Answer from the drawing. Dimensions are ordinates in mm from the lowest x, y and z of the part. Give positions to 0.01 mm unless a question says otherwise; leave off trailing zeros. Write each loop counter-clockwise with the first axis right and the second up, starting at its lowest first coordinate (ties: lowest second). Pieces come first, ordered by that corner, then holes. Notation, with made-up numbers: (-28.5, 29.5) - (29.5, 29.5) arc R28 cw to (29.5, 48.5) - close; hole circle Ø9 at (78.5, 83). An arc over 180 degrees is marked (long way). Answer as a JSON object with one key per item and string values. Group by question number.
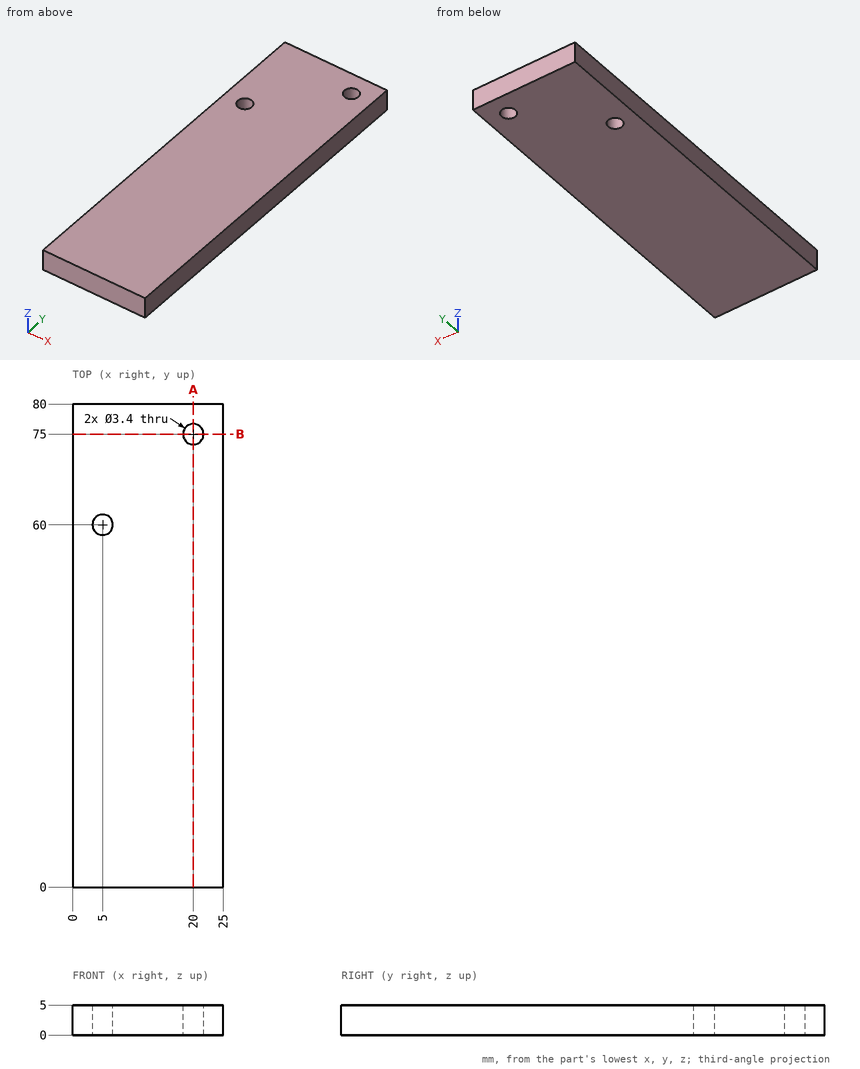
1) Find section A-A, the plane x = 20. Write down the section's boundary in (y, z), and give its area (3 significant figures).
2) Find the intervals of material crossed by line 1 (X direction, y = 75, z = 3.85); line 2 (Y direction, x = 20, z = 1.65); line 3 (Y direction, x = 5, z = 1.4), in increasing order. Write a range as [from, to].
3) Find section B-B, the plane y = 75. Write down the section's boundary in (x, z), and give its area (3 significant figures).
Values follow:
{
 "1": {"outline": "(0, 0) - (73.3, 0) - (73.3, 5) - (0, 5) - close; (76.7, 0) - (80, 0) - (80, 5) - (76.7, 5) - close", "area": "383 mm2"},
 "2": {"line 1": "x = [0, 18.3], [21.7, 25]", "line 2": "y = [0, 73.3], [76.7, 80]", "line 3": "y = [0, 58.3], [61.7, 80]"},
 "3": {"outline": "(0, 0) - (18.3, 0) - (18.3, 5) - (0, 5) - close; (21.7, 0) - (25, 0) - (25, 5) - (21.7, 5) - close", "area": "108 mm2"}
}
